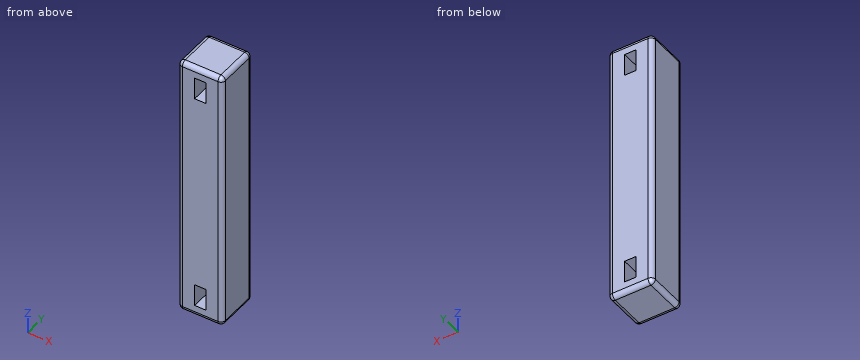
from build123d import *

# Parameters (mm, degrees)
F0_W     = 50.8
F0_H     = 304.8
F1_DEPTH = 25.4
F2_R     = 5.08
F3_W     = 12.7
F3_H     = 25.4
F4_DEPTH = 50.801
F5_W     = 12.7
F5_H     = 25.4
F6_DEPTH = 50.801


with BuildPart() as f1:
    # F0 (on Front) → F1 (new body, symmetric)
    with BuildSketch(Plane.XZ):
        with Locations((-0.276533, 53.275813)):
            Rectangle(F0_W, F0_H)
    extrude(amount=F1_DEPTH, both=True)

    # F2
    f2_edges = [f1.edges().sort_by_distance(p)[0] for p in [
        (25.123467, -25.4, 53.275813),
        (25.123467, 25.4, 53.275813),
        (-25.676533, 25.4, 53.275813),
        (-25.676533, -25.4, 53.275813),
        (25.123467, 0, 205.675813),
        (-0.276533, 25.4, 205.675813),
        (-25.676533, 0, 205.675813),
        (-0.276533, -25.4, 205.675813),
        (-0.276533, 25.4, -99.124187),
        (25.123467, 0, -99.124187),
        (-0.276533, -25.4, -99.124187),
        (-25.676533, 0, -99.124187),
    ]]
    fillet(f2_edges, radius=F2_R)

    # F3 (on face) → F4 (cut, through all)
    with BuildSketch(Plane.XZ.offset(25.4)):
        with Locations((-0.276533, 180.275813)):
            Rectangle(F3_W, F3_H)
    extrude(amount=-F4_DEPTH, mode=Mode.SUBTRACT)

    # F5 (on face) → F6 (cut, through all)
    with BuildSketch(Plane.XZ.offset(25.4)):
        with Locations((-0.276533, -73.724187)):
            Rectangle(F5_W, F5_H)
    extrude(amount=-F6_DEPTH, mode=Mode.SUBTRACT)


solid = f1.part
The model under review builds one solid part; all positions refer to its coordinate system, in mm. Round coordinates to 2 decimals unless told otherwise and drop trailing zeros. Loops run counter-clockwise (first coordinate to the right, second up) from the corner with the lowest first, then second, coordinate; pieces in that order, holes last. Notation, with made-up numbers: (3, 27.5) -> (17, 27.5) arc R15 cw to (17, 38.5) -> close; hole circle Ø5 at (14.25, 88.25). An arc over 180 degrees is marked (long way). Return JSON: item names as keys, results as strings.
(1) Add section B-B on y = 15.5. Write out the cut boundary in (x, z).
Solved:
{"outline": "(-25.68, -94.04) arc R5.08 ccw to (-20.6, -99.12) -> (20.04, -99.12) arc R5.08 ccw to (25.12, -94.04) -> (25.12, 200.6) arc R5.08 ccw to (20.04, 205.68) -> (-20.6, 205.68) arc R5.08 ccw to (-25.68, 200.6) -> close; hole (-6.63, -86.42) -> (6.07, -86.42) -> (6.07, -61.02) -> (-6.63, -61.02) -> close; hole (-6.63, 167.58) -> (6.07, 167.58) -> (6.07, 192.98) -> (-6.63, 192.98) -> close"}
(2) For line 1 (X direction, y = 2, z = 180.5); line 2 (Z direction, x = 3.5, y = -7); line 3 (Y direction, x = -21, z = 60), list the stretches that pass through material, from the lowest coordinate up.
Solved:
{"line 1": "-25.68 to -6.63, 6.07 to 25.12", "line 2": "-99.12 to -86.42, -61.02 to 167.58, 192.98 to 205.68", "line 3": "-25.38 to 25.38"}
(3) Add section A-A on x = 0. Write out the cut boundary in (y, z).
Solved:
{"outline": "(-25.4, -94.04) arc R5.08 ccw to (-20.32, -99.12) -> (20.32, -99.12) arc R5.08 ccw to (25.4, -94.04) -> (25.4, -86.42) -> (-25.4, -86.42) -> close; (-25.4, -61.02) -> (25.4, -61.02) -> (25.4, 167.58) -> (-25.4, 167.58) -> close; (-25.4, 192.98) -> (25.4, 192.98) -> (25.4, 200.6) arc R5.08 ccw to (20.32, 205.68) -> (-20.32, 205.68) arc R5.08 ccw to (-25.4, 200.6) -> close"}
